from build123d import *

# Parameters (mm, degrees)
F0_W         = 50.8
F0_H         = 50.8
F1_DEPTH     = 50.8
F2_R         = 5.08
F3_R         = 5.08
F4_T1_DEPTH  = 58.42
F4_T3_DEPTH  = 76.2
F4_T5_DEPTH  = 40.64
F4_S9_W      = 5.08
F4_S9_H      = 5.08
F4_T10_DEPTH = 5.08
F4_S15_W     = 5.08
F4_S15_H     = 5.08
F4_T16_DEPTH = 5.08
F4_T20_ANGLE = 90
F4_T22_ANGLE = 90
F5_T1_DEPTH  = 66.04
F6_T1_DEPTH  = 66.04
F7_R         = 3.81
F8_DEPTH     = 1.27


# Not quite as in the source:
# - a fillet or chamfer that OpenCascade refuses, or shapes differently, is made with other operations: its cross-section is extruded or revolved along the edge and cut away or added


with BuildPart() as f1:
    # F0 (on Front) → F1 (new body)
    with BuildSketch(Plane.XZ):
        with Locations((25.4, 25.4)):
            Rectangle(F0_W, F0_H)
    extrude(amount=F1_DEPTH)

    # F2
    f2_edges = [f1.edges().sort_by_distance(p)[0] for p in [
        (25.4, -50.8, 50.8),
    ]]
    fillet(f2_edges, radius=F2_R)

    # F3
    f3_edges = [f1.edges().sort_by_distance(p)[0] for p in [
        (25.4, 0, 50.8),
        (0, 0, 25.4),
        (25.4, 0, 0),
        (50.8, 0, 25.4),
    ]]
    fillet(f3_edges, radius=F3_R)

    # F4: fillet of radius 5.08 on 4 edges, made by hand

    # F4_s2 → F4_t1 (cut)
    with BuildSketch(Plane.XY.offset(-12.7)):
        with BuildLine():
            ThreePointArc((0, -45.72), (1.4878975516, -49.3121024484), (5.08, -50.8))
            Line((5.08, -50.8), (0, -50.8))
            Line((0, -50.8), (0, -45.72))
        make_face()
        with BuildLine():
            ThreePointArc((45.72, -50.8), (49.3121024484, -49.3121024484), (50.8, -45.72))
            Line((50.8, -45.72), (50.8, -50.8))
            Line((50.8, -50.8), (45.72, -50.8))
        make_face()
    extrude(amount=F4_T1_DEPTH, mode=Mode.SUBTRACT)

    # F4_s4 → F4_t3 (cut)
    with BuildSketch(Plane.YZ.offset(-12.7)):
        with BuildLine():
            ThreePointArc((-45.72, 0), (-49.3121024484, 1.4878975516), (-50.8, 5.08))
            Line((-50.8, 5.08), (-50.8, 0))
            Line((-50.8, 0), (-45.72, 0))
        make_face()
    extrude(amount=F4_T3_DEPTH, mode=Mode.SUBTRACT)

    # F4_s6 → F4_t5 (cut)
    with BuildSketch(Plane.XZ.offset(5.08)):
        with BuildLine():
            ThreePointArc((45.72, 50.8), (49.3121024484, 49.3121024484), (50.8, 45.72))
            Line((50.8, 45.72), (50.8, 50.8))
            Line((50.8, 50.8), (45.72, 50.8))
        make_face()
        with BuildLine():
            ThreePointArc((0, 45.72), (1.4878975516, 49.3121024484), (5.08, 50.8))
            Line((5.08, 50.8), (0, 50.8))
            Line((0, 50.8), (0, 45.72))
        make_face()
    extrude(amount=F4_T5_DEPTH, mode=Mode.SUBTRACT)


with BuildPart() as f4_tool8:
    # F4_s9 → F4_t10 (new body)
    with BuildSketch(Plane.XY.offset(45.72)):
        with Locations((48.26, -2.54)):
            Rectangle(F4_S9_W, F4_S9_H)
    extrude(amount=F4_T10_DEPTH)

    # F4_s11 → F4_t12 (revolve, cut)
    with BuildSketch(Plane(origin=(45.72, -5.08, 45.72), x_dir=(-0.7071067812, -0.7071067812, 0), z_dir=(-0.7071067812, 0.7071067812, 0))):
        with BuildLine():
            ThreePointArc((0, -5.08), (5.08, 0), (0, 5.08))
            Line((0, 5.08), (0, -5.08))
        make_face()
    revolve(axis=Axis((45.72, -5.08, 45.72), (0, 0, 1)), mode=Mode.SUBTRACT)


with BuildPart() as f1_1:
    add(f1.part)

    # F4_t7: cut F4_tool8
    add(f4_tool8.part, mode=Mode.SUBTRACT)


with BuildPart() as f4_tool14:
    # F4_s15 → F4_t16 (new body)
    with BuildSketch(Plane.YZ.offset(5.08)):
        with Locations((-2.54, 48.26)):
            Rectangle(F4_S15_W, F4_S15_H)
    extrude(amount=-F4_T16_DEPTH)

    # F4_s17 → F4_t18 (revolve, cut)
    with BuildSketch(Plane(origin=(5.08, -5.08, 45.72), x_dir=(0, -0.7071067812, -0.7071067812), z_dir=(0, 0.7071067812, -0.7071067812))):
        with BuildLine():
            ThreePointArc((0, -5.08), (5.08, 0), (0, 5.08))
            Line((0, 5.08), (0, -5.08))
        make_face()
    revolve(axis=Axis((5.08, -5.08, 45.72), (-1, 0, 0)), mode=Mode.SUBTRACT)


with BuildPart() as f1_2:
    add(f1_1.part)

    # F4_t13: cut F4_tool14
    add(f4_tool14.part, mode=Mode.SUBTRACT)

    # F4_s19 → F4_t20 (revolve, cut)
    with BuildSketch(Plane.XZ.offset(45.72)):
        with BuildLine():
            ThreePointArc((45.72, 50.8), (49.3121024484, 49.3121024484), (50.8, 45.72))
            Line((50.8, 45.72), (50.8, 50.8))
            Line((50.8, 50.8), (45.72, 50.8))
        make_face()
    revolve(axis=Axis((50.8, -45.72, 45.72), (1, 0, 0)), revolution_arc=F4_T20_ANGLE, mode=Mode.SUBTRACT)

    # F4_s21 → F4_t22 (revolve, cut)
    with BuildSketch(Plane.XZ.offset(45.72)):
        with BuildLine():
            ThreePointArc((0, 45.72), (1.4878975516, 49.3121024484), (5.08, 50.8))
            Line((5.08, 50.8), (0, 50.8))
            Line((0, 50.8), (0, 45.72))
        make_face()
    revolve(axis=Axis((0, -45.72, 45.72), (1, 0, 0)), revolution_arc=F4_T22_ANGLE, mode=Mode.SUBTRACT)

    # F5: fillet of radius 5.08 on 4 edges, made by hand

    # F5_s2 → F5_t1 (cut)
    with BuildSketch(Plane.XZ.offset(-7.62)):
        with BuildLine():
            ThreePointArc((0, 5.08), (1.4878975516, 1.4878975516), (5.08, 0))
            Line((5.08, 0), (0, 0))
            Line((0, 0), (0, 5.08))
        make_face()
    extrude(amount=F5_T1_DEPTH, mode=Mode.SUBTRACT)

    # F6: fillet of radius 5.08 on 4 edges, made by hand

    # F6_s2 → F6_t1 (cut)
    with BuildSketch(Plane.XZ.offset(-7.62)):
        with BuildLine():
            ThreePointArc((45.72, 0), (49.3121024484, 1.4878975516), (50.8, 5.08))
            Line((50.8, 5.08), (50.8, 0))
            Line((50.8, 0), (45.72, 0))
        make_face()
    extrude(amount=F6_T1_DEPTH, mode=Mode.SUBTRACT)

    # F7 (on face) → F8 (cut)
    with BuildSketch(Plane.YZ.offset(50.8)):
        with Locations((-25.4, 25.4)):
            Circle(F7_R)
    extrude(amount=-F8_DEPTH, mode=Mode.SUBTRACT)


solid = f1_2.part
Geometry: final body of the model. Coordinates: model frame, mm. Round coordinates to 2 decimals unless told otherwise and drop trailing zeros. Write each loop counter-clockwise with the first axis right and the second up, starting at its lowest first coordinate (ties: lowest second). Pieces come first, ordered by that corner, then holes. Notation, with made-up numbers: M 4,-17.5 L 31,-17.5 A26 cw 31,6.5 Z; hole C 72.25,5.25 d7. An arc over 180 degrees is marked long. Write item = value, one per line.
Item 1: Section query B-B on x = 47. Return loops of the section in (y, z), then the cut area to 3 significant figures.
Findings:
outline = M -50.64,3.8 A5.08 ccw -47,0.16 L -3.8,0.16 A5.08 ccw -0.16,3.8 L -0.16,45.72 A4.92 ccw -5.08,50.64 L -45.72,50.64 A4.92 ccw -50.64,45.72 Z
area = 2,530 mm^2
Item 2: Material intervals for line 1 along Z through (x, y) = (50, -25.4); line 2 along Y through (x, z) = (42, 5); line 3 along Z through (x, y) = (50.4, -25.4), sorted ascending. Write a range as [from, to].
Findings:
line_1 = [2.34, 21.59], [29.21, 48.46]
line_2 = [-50.8, 0]
line_3 = [3.1, 21.59], [29.21, 47.7]
Item 3: Pull-direction query (Y, two-part tool) for faces 1 (the face through (25.684, -1.528, 49.351)), 2 (the face through (49.272, -49.351, 23.294)), 3 (the face through (1.449, -25.116, 49.272)), 4 (the face through (49.53, -25, 25)); classes: pulls with the +Y half, pulls with the -Y half, needs draft (parallel to the pull), parting line crosses it, or undercut.
Findings:
face_1 = pulls with the +Y half
face_2 = pulls with the -Y half
face_3 = needs draft
face_4 = undercut
Item 4: Section query A-A on y = -4. Return loops of the section in (x, z).
Findings:
outline = M 0.12,4 A5.08 ccw 4,0.12 L 46.8,0.12 A5.08 ccw 50.68,4 L 50.68,45.72 A4.96 ccw 45.72,50.68 L 5.08,50.68 A4.96 ccw 0.12,45.72 Z
Item 5: Pin query (flat end, axial travel): P1, Ø2.5, axis at y = -25.5, z = 26.5, coming from the +X side. Return the tip coordinate at first contact, or that it passes through.
Findings:
P1 = 49.53
